Model file for the job. Use its own axes, mm. Give positions to 0.01 mm unless a question says otherwise; leave off trailing zeros. Loops run counter-clockwise (first coordinate to the right, second up) from the corner with the lowest first, then second, coordinate; pieces in that order, holes last. Notation, with made-up numbers: M 63.5,47 L 107.5,47 A28 cw 107.5,65 Z; hole C -24.5,15.25 d4. An arc over 180 degrees is marked long. Answer in a Markdown table with one row per item.
```python
from build123d import *

# Parameters (mm, degrees)
CYLINDER_R         = 3.15
CYLINDER_DEPTH     = 13
BOX009_W           = 6
BOX009_H           = 24
BOX009_DEPTH       = 16
CHAMFER020020_SIZE = 3


with BuildPart() as cylinder:
    # Cylinder → Cylinder (new body)
    with BuildSketch(Plane(origin=(0, 15, -14), x_dir=(0, 0, -1), z_dir=(1, 0, 0))):
        Circle(CYLINDER_R)
    extrude(amount=CYLINDER_DEPTH)


with BuildPart() as cut002002002007004004001004:
    # Box009 → Box009 (new body)
    with BuildSketch(Plane(origin=(0, 3, -22), x_dir=(1, 0, 0), z_dir=(0, 0, 1))):
        with Locations((3, 12)):
            Rectangle(BOX009_W, BOX009_H)
    extrude(amount=BOX009_DEPTH)

    # Chamfer020020
    chamfer020020_edges = [cut002002002007004004001004.edges().sort_by_distance(p)[0] for p in [
        (3, 3, -22),
        (3, 27, -22),
    ]]
    chamfer(chamfer020020_edges, length=CHAMFER020020_SIZE)

    # Cut002002002007004004001004: cut Cylinder
    add(cylinder.part, mode=Mode.SUBTRACT)


solid = cut002002002007004004001004.part
```
(1) Saw through at A-A, the plane z = -14. Give the cut face in (x, y).
Established:
| item | result |
|---|---|
| outline | M 0,3 L 6,3 L 6,11.85 L 0,11.85 Z; M 0,18.15 L 6,18.15 L 6,27 L 0,27 Z |
(2) Saw through at B-B, the plane y = 16. Give the cut face in (x, z), and give its area (3 significant figures).
Established:
| item | result |
|---|---|
| outline | M 0,-22 L 6,-22 L 6,-16.99 L 0,-16.99 Z; M 0,-11.01 L 6,-11.01 L 6,-6 L 0,-6 Z |
| area | 60.2 mm2 |
(3) Mould opens along Y. For faces 1 (the cylindrical face through (2.958, 13.083, -11.5)), 2 (the flat face through (3, 27, -13)), 3 (the flat face through (3, 15, -6)) say: pulls with the +Y half, pulls with the -Y half, needs draft (parallel to the pull), parting line crosses it, or undercut.
Established:
| item | result |
|---|---|
| face 1 | undercut |
| face 2 | pulls with the +Y half |
| face 3 | needs draft |
(4) Saw through at C-C, the plane x = 0.8. Give the cut face in (y, z).
Established:
| item | result |
|---|---|
| outline | M 3,-19 L 6,-22 L 24,-22 L 27,-19 L 27,-6 L 3,-6 Z; hole C 15,-14 d6.3 |
(5) Wall check: L1, parallel to Z at x = 3.7, y = 15; L2, parallel to Y at x = 1.9, z = -14; L3, parallel to Y at x = 1.3, z = -15.75. Give the ranges that are in metal, low to high.
Established:
| item | result |
|---|---|
| L1 | z = -22 to -17.15, -10.85 to -6 |
| L2 | y = 3 to 11.85, 18.15 to 27 |
| L3 | y = 3 to 12.38, 17.62 to 27 |
